Read the model definition and answer for the solid it produces. Units are mm, in the model's axes. Face numbers are marked on the shaded views. Give positions to 0.01 mm unless a question says otherwise; leave off trailing zeros. Write each loop counter-clockwise with the first axis right and the second up, starting at its lowest first coordinate (ties: lowest second). Pieces come first, ordered by that corner, then holes. Notation, with made-up numbers: (-35.75, 63) - (-31.75, 63) arc R7 cw to (-31.75, 72) - close; hole circle Ø6 at (83, -24). An arc over 180 degrees is marked (long way). Use CSV: the item, a comma, the result in double quotes. Start each with the question number.
Autodesk Inventor part; units mm, degrees
ref_plane "YZ Plane" through (0, 0, 0) normal (1, 0, 0) x (0, 1, 0)
ref_plane "XZ Plane" through (0, 0, 0) normal (0, 1, 0) x (-1, 0, 0)
ref_plane "XY Plane" through (0, 0, 0) normal (0, 0, 1) x (1, 0, 0)
sketch "Sketch_1" plane through (0, 0, 0) normal (1, 0, 0) x (0, 1, 0)
  line L0 (2.3431, 50) -> (0, 50)
  line L1 (0, 50) -> (0, 0)
  line L2 (0, 0) -> (50, 0)
  line L3 (50, 0) -> (50, 2.3431)
  arc A0 (50, 2.3431) -> (48.8284, 5.1716) centre (46, 2.3431) ccw
  line L4 (48.8284, 5.1716) -> (5.1716, 48.8284)
  arc A1 (5.1716, 48.8284) -> (2.3431, 50) centre (2.3431, 46) ccw
  line L5 (4, 44.3431) -> (4, 4)
  line L6 (4, 4) -> (44.3431, 4)
  line L7 (44.3431, 4) -> (4, 44.3431)
extrude "Extrusion1" add sketch "Sketch_1" along normal mid plane 22
sketch "Sketch2" plane through (-11, 0, 0) normal (0, -1, 0) x (1, 0, 0)
  point P0 (11, 12.5)
hole "Hole1" at (0, 0, 12.5) direction (0, 1, 0) diameter 6.81 depth 4
sketch "Sketch3" plane through (11, 50, 0) normal (0, 0, -1) x (-1, 0, 0)
  point P0 (11, -37.5)
hole "Hole2" at (0, 12.5, 0) direction (0, 0, 1) diameter 6.81 depth 4
sketch "Sketch_4" plane through (0, 0, 50) normal (0, 0, 1) x (1, 0, 0)
  circle A0 centre (0, 12.5) radius 6.35
extrude "Extrusion2" cut sketch "Sketch_4" against normal blind 46
sketch "Sketch_5" plane through (0, 50, 0) normal (0, 1, 0) x (1, 0, 0)
  circle A0 centre (0, -12.5) radius 6.35
extrude "Extrusion3" cut sketch "Sketch_5" against normal blind 46
sketch "Sketch6" plane through (11, 50, 0) normal (0, 0, -1) x (-1, 0, 0)
  point P0 (11, -12.5)
hole "Hole3" at (0, 37.5, 0) direction (0, 0, 1) diameter 6.81 depth 4
sketch "Sketch7" plane through (-11, 0, 0) normal (0, -1, 0) x (1, 0, 0)
  point P0 (11, 37.5)
hole "Hole4" at (0, 0, 37.5) direction (0, 1, 0) diameter 6.81 depth 4
sketch "Sketch_8" plane through (0, 0, 50) normal (0, 0, 1) x (1, 0, 0)
  circle A0 centre (0, 37.5) radius 6.35
extrude "Extrusion4" cut sketch "Sketch_8" against normal blind 46
sketch "Sketch_9" plane through (0, 50, 0) normal (0, 1, 0) x (1, 0, 0)
  circle A0 centre (0, -37.5) radius 6.35
extrude "Extrusion5" cut sketch "Sketch_9" against normal blind 46
properties part number "25-4136 Aluminum"
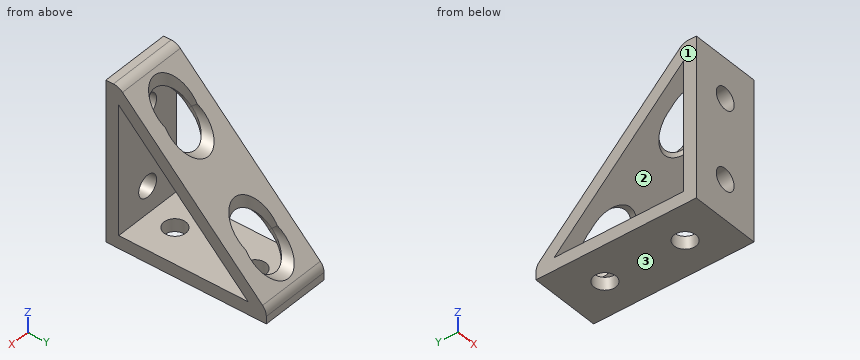
(1) For a pull along Z with two mould halves and no side action, classify the marked faces 1, 2 and 3 as pulls with the +Z half, pulls with the -Z half, needs draft (parallel to the pull), parting line crosses it, or undercut.
(2) The part is cut by section C-C on y = 42.5. Write down the section's boundary in (x, z).
(3) The part is cut by section B-B on z = 7. Write down the section's boundary in (x, y) (3 decimals).
(4) Given P1, Ø6.5, axis at x = 3.5, z = 32, coming from the +Y side; P2, Ø9, axis at x = 0, y = 37.5, coming from the +Z side; P3, Ø10, axis at x = 0, z = 37.5, coming from the +Y side, each flat-ended and moving along its own axis, determine where each tip first touches the part or whether it passes through.
(5) The part is cut by section D-D on x = 0. Give the number of separate pieces and of enclosed holes in the cut face, plus the area to 3 significant figures.
(6) Consider probe 1 along Y at (x, z) = (0, 1.25) (3 decimals); probe 2 along Y at (x, z) = (-3, 3); probe 3 along X at (y, z) = (12.5, 1.7) (3 decimals). Determine where each line is inside the solid, lowest interval first.
(7) The part is cut by section A-A on x = -7.5. Write down the section's boundary in (y, z), plus the area to 3 significant figures.
Reported:
1,face 1,"needs draft"
1,face 2,"undercut"
1,face 3,"pulls with the -Z half"
2,outline,"(-11, 0) - (11, 0) - (11, 4) - (-11, 4) - close; (-11, 5.84) - (-3.91, 5.84) - (-3.91, 7.5) arc R6.35 cw to (-6.27, 11.5) - (-11, 11.5) - close; (3.91, 5.84) - (11, 5.84) - (11, 11.5) - (6.27, 11.5) arc R6.35 cw to (3.91, 7.5) - close"
3,outline,"(-11, 0) - (11, 0) - (11, 4) - (-11, 4) - close; (-11, 41.343) - (-5.055, 41.343) arc R6.35 cw to (-3.174, 43) - (-3.174, 47) - (-11, 47) - close; (3.174, 43) arc R6.35 cw to (5.055, 41.343) - (11, 41.343) - (11, 47) - (3.174, 47) - close"
4,P1,"y = 25.25"
4,P2,"z = 4"
4,P3,"y = 4"
5,separate pieces,"6"
5,enclosed holes,"0"
5,area,"356 mm²"
6,probe 1,"0 to 9.095, 15.905 to 34.095, 40.905 to 50"
6,probe 2,"0 to 10.89, 14.11 to 35.89, 39.11 to 49.95"
6,probe 3,"-11 to -3.405, 3.405 to 11"
7,outline,"(0, 0) - (50, 0) - (50, 2.34) arc R4 ccw to (48.83, 5.17) - (5.17, 48.83) arc R4 ccw to (2.34, 50) - (0, 50) - close; hole (4, 4) - (44.34, 4) - (4, 44.34) - close"
7,area,"628 mm²"
